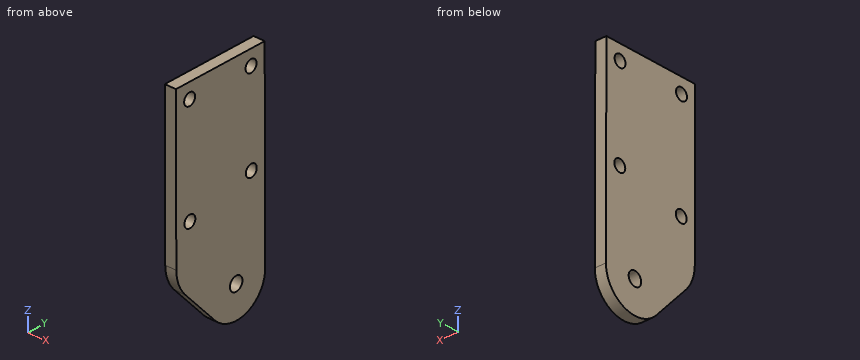
from build123d import *

# Parameters (mm, degrees)
SKETCH_1_R      = 1.839883841
SKETCH_1_R_2    = 1.6
EXTRUDE_1_DEPTH = 3


with BuildPart() as part:
    # 草图1 → 凸台-拉伸1 (new body)
    with BuildSketch(Plane(origin=(0, 0, 0), x_dir=(0, 0, -1), z_dir=(1, 0, 0))):
        with BuildLine():
            Line((-51.910708478, -17.756118332), (-10.410879829, -17.636861799))
            ThreePointArc((-10.410879829, -17.636861799), (-6.80853031, -16.954371319), (-3.69429735, -15.01936011))
            Line((-3.69429735, -15.01936011), (6.053738335, -6.112622142))
            ThreePointArc((6.053738335, -6.112622142), (7.885847556, 3.160295303), (0.014361881, 8.393204188))
            Line((0.014361881, 8.393204188), (-51.985423414, 8.243774315))
            Line((-51.985423414, 8.243774315), (-51.910708478, -17.756118332))
        make_face()
        with Locations((0.038787918, -0.106760716)):
            Circle(SKETCH_1_R, mode=Mode.SUBTRACT)
        with Locations((-47.973945324, 4.255285437)):
            Circle(SKETCH_1_R_2, mode=Mode.SUBTRACT)
        with Locations((-19.92233521, -13.664178003)):
            Circle(SKETCH_1_R_2, mode=Mode.SUBTRACT)
        with Locations((-23.974044419, 4.32425307)):
            Circle(SKETCH_1_R_2, mode=Mode.SUBTRACT)
        with Locations((-47.922219599, -13.744640242)):
            Circle(SKETCH_1_R_2, mode=Mode.SUBTRACT)
    extrude(amount=EXTRUDE_1_DEPTH)


solid = part.part
The listing builds one solid part. Answer for the finished solid, in the listing's coordinates (mm). Give positions to 0.01 mm unless a question says otherwise; leave off trailing zeros. Write each loop counter-clockwise with the first axis right and the second up, starting at its lowest first coordinate (ties: lowest second). Pieces come first, ordered by that corner, then holes. Notation, with made-up numbers: (9.25, -25.75) -> (47.25, -25.75) arc R14 ccw to (47.25, -3.75) -> close; hole circle Ø5 at (-13.75, 45.5). An arc over 180 degrees is marked (long way). One line per question, with ' | ' between items. Start each with the question number.
1. Section D-D (y = -11.25) is taken. Determine the outline of the cut face in (x, z).
2. Section A-A (y = -0.75) is taken. Determine the outline of the cut face in (x, z) (3 decimals), plus the area to 3 significant figures.
3. Given pin 1 Ø1.9 at (y, z) = (-13.66, 19.92) entering from -X; pin 2 Ø1 at (y, z) = (2, 26) entering from -X, each flat-ended and moving along its own axis, determine where each tip first touches the part or whether it passes through.
4. Section C-C (y = -5.5) is taken. Determine the outline of the cut face in (x, z), plus the area to 3 significant figures.
5. Find the intervals of material crossed by probe 1 along Z at (x, y) = (1.3, -14.25); probe 2 along Y at (x, z) = (1.1, 25); probe 3 along Y at (x, z) = (0.7, 18.5), in increasing order.
6. Section B-B (x = 1) is taken. Determine the outline of the cut face in (y, z), plus the area to 3 significant figures.
Response values:
1) outline: (0, -0.43) -> (3, -0.43) -> (3, 51.93) -> (0, 51.93) -> close
2) outline: (0, -8.514) -> (3, -8.514) -> (3, -1.763) -> (0, -1.763) -> close; (0, 1.685) -> (3, 1.685) -> (3, 51.96) -> (0, 51.96) -> close | area: 171 mm2
3) pin 1: through | pin 2: x = 0
4) outline: (0, -6.61) -> (3, -6.61) -> (3, 51.95) -> (0, 51.95) -> close | area: 176 mm2
5) probe 1: 2.85 to 18.43, 21.41 to 46.4, 49.44 to 51.92 | probe 2: -17.68 to 3.1, 5.55 to 8.32 | probe 3: -17.66 to -14.4, -12.93 to 8.34
6) outline: (-17.76, 51.91) -> (-17.64, 10.41) arc R10 ccw to (-15.02, 3.69) -> (-6.11, -6.05) arc R8.5 ccw to (8.39, -0.01) -> (8.24, 51.99) -> close; hole circle Ø3.2 at (-13.74, 47.92); hole circle Ø3.2 at (-13.66, 19.92); hole circle Ø3.68 at (-0.11, -0.04); hole circle Ø3.2 at (4.26, 47.97); hole circle Ø3.2 at (4.32, 23.97) | area: 1,410 mm2
